For this review, use the dimensioned drawing (mm, ordinates from the lowest corner) and the shaded views. A direction names the side the tool comes from. Coordinates: 2 decimals unless noted, no trailing zeros. Write each loop counter-clockwise with the first axis right and the second up, starting at its lowest first coordinate (ties: lowest second). Pieces come first, ordered by that corner, then holes. Notation, with made-up numbers: (60, 71) - (69, 71) arc R19 cw to (69, 83) - close; hole circle Ø2 at (48, 83). An arc over 180 degrees is marked (long way). Use one line per item in the form item = value. Start each with the question number.
1) We need section D-D (z = 13.5). Give the boundary of the cut face in (x, y) (3 decimals), plus the area to 3 significant figures.
2) We need section A-A (y = 2.25). Give the boundary of the cut face in (x, z) (3 decimals).
3) Tool access review of the marked faces 1, 2 and 3: name each direction out of +Z, -Z, +X, -X, +Y, -Y from which nothing blocks a thin tool from reaching the whole face with its end or side.
4) We need section C-C (z = 7.5). Give the boundary of the cut face in (x, y).
5) Insertion check: P1, Ø1, axis at x = 1, y = 3.5, coming from the -Z side; P2, Ø1.5, axis at y = 1.5, z = 2.5, coming from the +X side (3 decimals). Each pin has a flat end and moves straight along its axis. Give the tip position at first contact, or say it passes through.
6) For L1, parallel to Z at x = 0.25, y = 1.3; L2, parallel to Y at x = 1.95, z = 9.75; L3, parallel to X at y = 1.6, z = 12.5, list the stretches that pass through material, from the lowest coordinate up. Write a range as from..to.
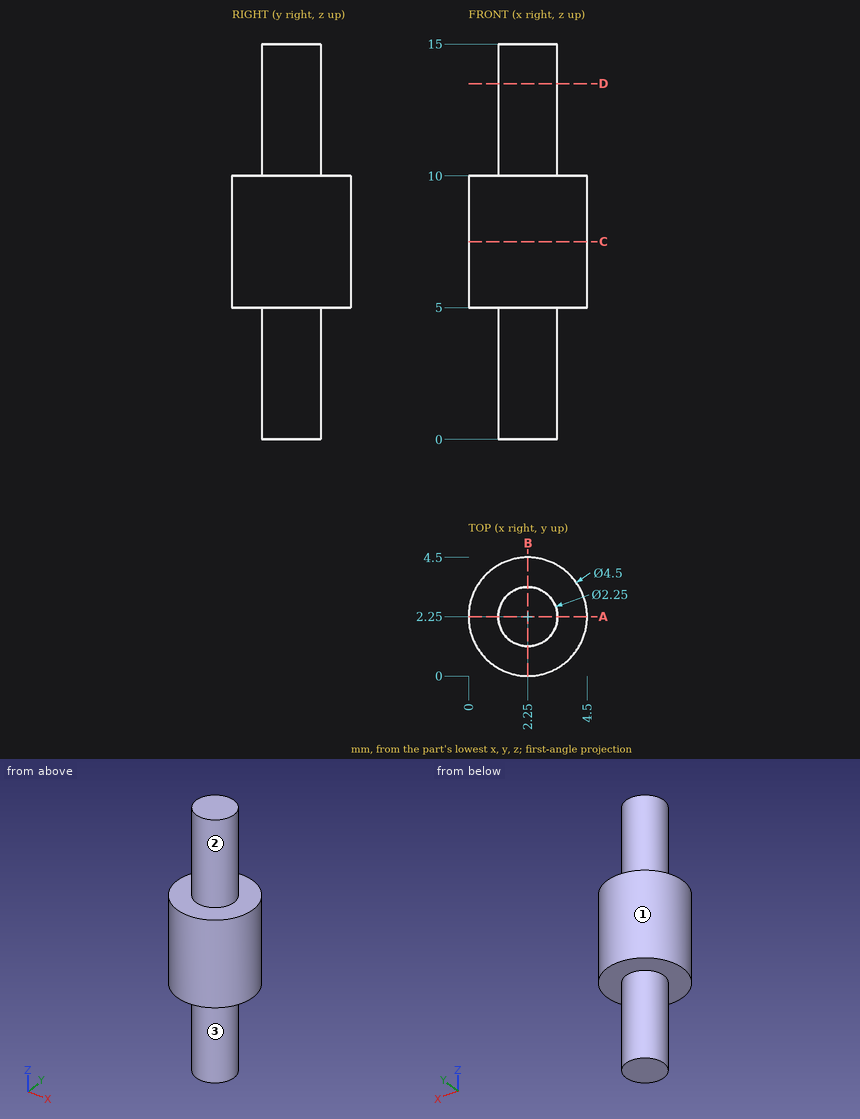
Determined:
q1.outline = circle Ø2.25 at (2.25, 2.25)
q1.area = 3.98 mm²
q2.outline = (0, 5) - (1.125, 5) - (1.125, 0) - (3.375, 0) - (3.375, 5) - (4.5, 5) - (4.5, 10) - (3.375, 10) - (3.375, 15) - (1.125, 15) - (1.125, 10) - (0, 10) - close
q3.face_1 = +Z, -Z
q3.face_2 = +Z
q3.face_3 = -Z
q4.outline = circle Ø4.5 at (2.25, 2.25)
q5.P1 = 5
q5.P2 = 3.375
q6.L1 = 5..10
q6.L2 = 0.02..4.48
q6.L3 = 1.33..3.17
